```python
from build123d import *

# Parameters (mm, degrees)
SKETCH1_R             = 65
SKETCH1_R_2           = 5
SKETCH1_R_3           = 12.5
BOSS_EXTRUDE1_DEPTH   = 10
SKETCH2_R             = 24
SKETCH2_R_2           = 12.5
BOSS_EXTRUDE2_DEPTH   = 20
CHAMFER1_SIZE         = 1
FILLET1_R             = 3
CHAMFER2_SIZE         = 1
SKETCH4_W             = 8
SKETCH4_H             = 16.3
CUT_EXTRUDE2_DEPTH    = 97.695398029
M5_TAPPED_HOLE1_D     = 4.2
M5_TAPPED_HOLE1_DEPTH = 12.4
M5_TAPPED_HOLE1_TIP   = 1.2618073


with BuildPart() as part:
    # Sketch1 → Boss-Extrude1 (new body)
    with BuildSketch(Plane.XY):
        Circle(SKETCH1_R)
        with Locations((0, 55)):
            Circle(SKETCH1_R_2, mode=Mode.SUBTRACT)
        Circle(SKETCH1_R_3, mode=Mode.SUBTRACT)
    extrude(amount=BOSS_EXTRUDE1_DEPTH)

    # Sketch2 → Boss-Extrude2 (add)
    with BuildSketch(Plane.XY.offset(10)):
        Circle(SKETCH2_R)
        Circle(SKETCH2_R_2, mode=Mode.SUBTRACT)
    extrude(amount=BOSS_EXTRUDE2_DEPTH)

    # Chamfer1
    chamfer1_edges = [part.edges().sort_by_distance(p)[0] for p in [
        (-65, 0, 0),
        (-65, 0, 10),
    ]]
    chamfer(chamfer1_edges, length=CHAMFER1_SIZE)

    # Fillet1
    fillet1_edges = [part.edges().sort_by_distance(p)[0] for p in [
        (-24, 0, 10),
    ]]
    fillet(fillet1_edges, radius=FILLET1_R)

    # Chamfer2
    chamfer2_edges = [part.edges().sort_by_distance(p)[0] for p in [
        (-24, 0, 30),
    ]]
    chamfer(chamfer2_edges, length=CHAMFER2_SIZE)

    # Sketch4 → Cut-Extrude2 (cut, through all)
    with BuildSketch(Plane.XY.offset(30)):
        with Locations((0, 8.15)):
            Rectangle(SKETCH4_W, SKETCH4_H)
    extrude(amount=-CUT_EXTRUDE2_DEPTH, mode=Mode.SUBTRACT)

    # M5 Tapped Hole1
    with Locations(Plane(origin=(0, 16.3, 0), x_dir=(-1, 0, 0), z_dir=(0, -1, 0))):
        with Locations((0, -20)):
            Hole(M5_TAPPED_HOLE1_D / 2, depth=M5_TAPPED_HOLE1_DEPTH)
            with Locations((0, 0, -(M5_TAPPED_HOLE1_DEPTH + M5_TAPPED_HOLE1_TIP / 2))):  # 118° drill point
                Cone(0, M5_TAPPED_HOLE1_D / 2, M5_TAPPED_HOLE1_TIP, mode=Mode.SUBTRACT)


solid = part.part
```
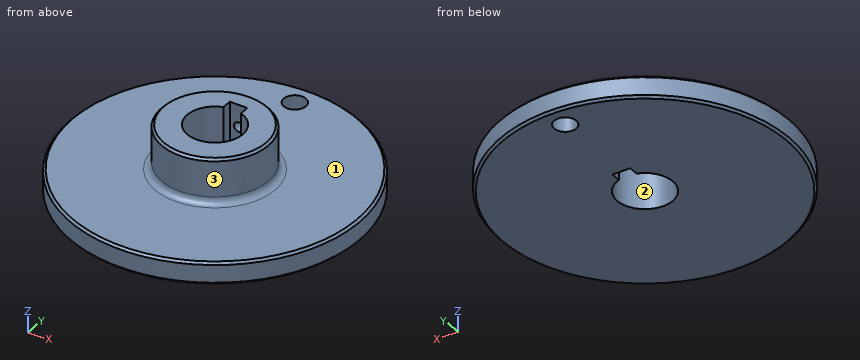
Check sheet for the modelled part. Datum: model origin and axes. Units: mm. Face numbers are marked on the shaded views. Round coordinates to 2 decimals unless told otherwise and drop trailing zeros. Write each loop counter-clockwise with the first axis right and the second up, starting at its lowest first coordinate (ties: lowest second). Pieces come first, ordered by that corner, then holes. Notation, with made-up numbers: (76.5, -6.5) -> (106.5, -6.5) arc R12 ccw to (106.5, 7.5) -> close; hole circle Ø3 at (53.25, -39.75). An arc over 180 degrees is marked (long way). Put each result on its own line as item: value.
(1) Sectioned sample at B-B (z = 15.75). Enter the section's corners in (x, y).
Values found:
outline: circle Ø48 at (0, 0); hole (-4, 11.84) arc R12.5 ccw (long way) to (4, 11.84) -> (4, 16.3) -> (-4, 16.3) -> close
(2) Go/stop test with flat-tipped pins: pin 1 Ø8 at (x, z) = (12.5, 13) entering from +Y; pin 2 Ø4 at (y, z) = (16.5, 13) entering from +X; pin 3 Ø3.5 at (y, z) = (15, 21) entering from -X. Record where each tip stops, or that it passes through.
Values found:
pin 1: stops at y = 63.86
pin 2: stops at x = 19.14
pin 3: stops at x = -20.01
(3) Sectioned sample at C-C (z = 4). Enter the section's corners in (x, y), plus the area to 3 significant figures.
Values found:
outline: circle Ø130 at (0, 0); hole circle Ø10 at (0, 55); hole (-4, 11.84) arc R12.5 ccw (long way) to (4, 11.84) -> (4, 16.3) -> (-4, 16.3) -> close
area: 12,700 mm^2
(4) Material ranges on line 1 (Y direction, x = 0, z = 7); line 2 (Z direction, x = 0, y = 22); line 3 (Z direction, x = -31.5, y = -11), recorded low to high.
Values found:
line 1: y = -65 to -12.5, 16.3 to 50, 60 to 65
line 2: z = 0 to 17.9, 22.1 to 30
line 3: z = 0 to 10
(5) Sectioned sample at A-A (x = 0). Enter the section's corners in (y, z).
Values found:
outline: (-65, 1) -> (-64, 0) -> (-12.5, 0) -> (-12.5, 30) -> (-23, 30) -> (-24, 29) -> (-24, 13) arc R3 cw to (-27, 10) -> (-64, 10) -> (-65, 9) -> close; (16.3, 0) -> (50, 0) -> (50, 10) -> (27, 10) arc R3 cw to (24, 13) -> (24, 17.9) -> (16.3, 17.9) -> close; (16.3, 22.1) -> (24, 22.1) -> (24, 29) -> (23, 30) -> (16.3, 30) -> close; (60, 0) -> (64, 0) -> (65, 1) -> (65, 9) -> (64, 10) -> (60, 10) -> close
(6) Mould release check, pull along Y, two halves, no side actions. Record for the marked faces 1, 2 and 3: released by +Y, released by -Y, zero draft, split by the parting line, or undercut.
Values found:
face 1: zero draft
face 2: undercut
face 3: split by the parting line
